from build123d import *

# Parameters (mm, degrees)
EXTRUDE_1_DEPTH             = 8
SKETCH_2_R                  = 2.5
EXTRUDE_2_DEPTH             = 6
SKETCH_3_R                  = 2.5
SKETCH_3_R_2                = 2.1
CUT_EXTRUDE_3_DEPTH         = 0.5
CHAMFER_1_SIZE              = 0.4
HOLE_WIZARD_M41_D           = 3.3
HOLE_WIZARD_M41_DEPTH       = 6
HOLE_WIZARD_M41_CSINK_D     = 4
HOLE_WIZARD_M41_CSINK_ANGLE = 90
HOLE_WIZARD_M41_TIP         = 0.991420021


with BuildPart() as part:
    # Эскиз1 → Вытянуть1 (new body)
    with BuildSketch(Plane.XY):
        Polygon((0, 4.041451884), (-3.5, 2.020725942), (-3.5, -2.020725942), (0, -4.041451884), (3.5, -2.020725942), (3.5, 2.020725942), align=None)
    extrude(amount=EXTRUDE_1_DEPTH)

    # Эскиз2 → Вытянуть2 (add)
    with BuildSketch(Plane.XY.offset(8)):
        Circle(SKETCH_2_R)
    extrude(amount=EXTRUDE_2_DEPTH)

    # Эскиз3 → Вырез-Вытянуть3 (cut)
    with BuildSketch(Plane.XY.offset(8)):
        Circle(SKETCH_3_R)
        Circle(SKETCH_3_R_2, mode=Mode.SUBTRACT)
    extrude(amount=CUT_EXTRUDE_3_DEPTH, mode=Mode.SUBTRACT)

    # Фаска1
    chamfer_1_edges = [part.edges().sort_by_distance(p)[0] for p in [
        (-2.5, 0, 8.5),
        (-2.5, 0, 14),
    ]]
    chamfer(chamfer_1_edges, length=CHAMFER_1_SIZE - 0.0001)  # a hair under: the kernel refuses the full size

    # Отверстие с зазором M41
    with Locations(Plane(origin=(0, 0, 0), x_dir=(-1, 0, 0), z_dir=(0, 0, -1))):
        with Locations((0, 0)):
            CounterSinkHole(HOLE_WIZARD_M41_D / 2, HOLE_WIZARD_M41_CSINK_D / 2, depth=HOLE_WIZARD_M41_DEPTH, counter_sink_angle=HOLE_WIZARD_M41_CSINK_ANGLE)
            with Locations((0, 0, -(HOLE_WIZARD_M41_DEPTH + HOLE_WIZARD_M41_TIP / 2))):  # 118° drill point
                Cone(0, HOLE_WIZARD_M41_D / 2, HOLE_WIZARD_M41_TIP, mode=Mode.SUBTRACT)


solid = part.part
CAD build for the part. Positions are in the model's coordinates, mm. A direction names the side the tool comes from. Give positions to 0.01 mm unless a question says otherwise; leave off trailing zeros. Write each loop counter-clockwise with the first axis right and the second up, starting at its lowest first coordinate (ties: lowest second). Pieces come first, ordered by that corner, then holes. Notation, with made-up numbers: (80.25, 71) - (129.25, 71) arc R10 ccw to (129.25, 85) - close; hole circle Ø11 at (2, -23). An arc over 180 degrees is marked (long way). Answer as CSV lines item,"result".
Q1. Band-saw the part on A-A (z = 2). Give the cut face in (x, y).
Result set:
outline,"(-3.5, -2.02) - (0, -4.04) - (3.5, -2.02) - (3.5, 2.02) - (0, 4.04) - (-3.5, 2.02) - close; hole circle Ø3.3 at (0, 0)"
Q2. Flat gauge pins, fed straight in: pin 1 Ø4 at (x, z) = (-2.5, 5) entering from +Y; pin 2 Ø1.5 at (x, z) = (-3, 12) entering from +Y; pin 3 Ø3 at (x, z) = (1, 1.5) entering from +Y. Where does each tip first touch, or does it go through?
Result set:
pin 1,"y = 3.75"
pin 2,"y = 1.09"
pin 3,"y = 4.04"
Q3. Drill centre lines: line 1 (X direction, y = 0, z = 1.8); line 2 (Z direction, x = 0.5, y = -2.5); line 3 (X direction, y = 1.5, z = 12.25). Where is each one in solid material? Low to high. Write a range as from..to.
Result set:
line 1,"-3.5..-1.65, 1.65..3.5"
line 2,"0..8"
line 3,"-2..2"
Q4. Pull direction Z, two halves, no side cores. Call faces 1 (the face through (3.5, 0, 4)), 2 (the face through (2.003, 0.631, 8.246)), 3 (the face through (-2, -2, 0)): released by +Z, released by -Z, zero draft, split by the parting line, or undercut.
Result set:
face 1,"zero draft"
face 2,"undercut"
face 3,"released by -Z"
Q5. 3-axis set-ups, long thin cutter, end or side, ignore diameter. For faces 4 (the face through (-2, -2, 8)), 5 (the face through (-1.216, 1.115, 3.215)), 6 (the face through (-1.726, 3.045, 3.944)), 7 (the face through (-0.54, -2.44, 11.22)), 8 (the face through (-3.5, 0, 4)): which of +Z, -Z, +X, -X, +Y, -Y reach the whole face in a straight line?
Result set:
face 4,"none"
face 5,"-Z"
face 6,"+Z, -Z, -X, +Y"
face 7,"+Z"
face 8,"+Z, -Z, -X, +Y, -Y"
Q6. Band-saw the part on B-B (y = 3.25). Give the cut face in (x, z), and give its area (3 significant figures).
Result set:
outline,"(-1.37, 0) - (1.37, 0) - (1.37, 8) - (-1.37, 8) - close"
area,"21.9 mm²"
